```python
from build123d import *

# Parameters (mm, degrees)
BOSS_EXTRUDE1_DEPTH = 15
BOSS_EXTRUDE2_DEPTH = 7.5
SKETCH3_W           = 40
SKETCH3_H           = 75
SKETCH3_R           = 1.5
BOSS_EXTRUDE3_DEPTH = 15


with BuildPart() as part:
    # Sketch1 → Boss-Extrude1 (new body)
    with BuildSketch(Plane(origin=(0, 0, 0), x_dir=(0, 0, -1), z_dir=(1, 0, 0))):
        with BuildLine():
            Line((-37.5, 34), (-37.5, 40))
            Line((-37.5, 40), (-75, 40))
            Line((-75, 40), (-75, 0))
            Line((-75, 0), (-37.5, 0))
            Line((-37.5, 0), (-37.5, 6))
            ThreePointArc((-37.5, 6), (-51.5, 20), (-37.5, 34))
        make_face()
        with BuildLine():
            Line((0, 40), (-37.5, 40))
            Line((-37.5, 40), (-37.5, 34))
            ThreePointArc((-37.5, 34), (-27.600505063, 29.899494937), (-23.5, 20))
            ThreePointArc((-23.5, 20), (-27.600505063, 10.100505063), (-37.5, 6))
            Line((-37.5, 6), (-37.5, 0))
            Line((-37.5, 0), (0, 0))
            Line((0, 0), (0, 40))
        make_face()
    extrude(amount=BOSS_EXTRUDE1_DEPTH)

    # Sketch1_3 → Boss-Extrude2 (add)
    with BuildSketch(Plane(origin=(0, 0, 0), x_dir=(0, 0, -1), z_dir=(1, 0, 0))):
        with BuildLine():
            ThreePointArc((-23.5, 20), (-27.600505063, 29.899494937), (-37.5, 34))
            Line((-37.5, 34), (-37.5, 23))
            ThreePointArc((-37.5, 23), (-35.378679656, 22.121320344), (-34.5, 20))
            ThreePointArc((-34.5, 20), (-35.378679656, 17.878679656), (-37.5, 17))
            Line((-37.5, 17), (-37.5, 6))
            ThreePointArc((-37.5, 6), (-27.600505063, 10.100505063), (-23.5, 20))
        make_face()
        with BuildLine():
            Line((-37.5, 23), (-37.5, 34))
            ThreePointArc((-37.5, 34), (-51.5, 20), (-37.5, 6))
            Line((-37.5, 6), (-37.5, 17))
            ThreePointArc((-37.5, 17), (-40.5, 20), (-37.5, 23))
        make_face()
    extrude(amount=BOSS_EXTRUDE2_DEPTH)

    # Sketch3 → Boss-Extrude3 (add)
    with BuildSketch(Plane(origin=(0, 40, 0), x_dir=(1, 0, 0), z_dir=(0, 1, 0))):
        with Locations((20, -37.5)):
            Rectangle(SKETCH3_W, SKETCH3_H)
        with Locations(Location((8.5, -17.25, 0), (0, 0, 270))):
            Circle(SKETCH3_R, mode=Mode.SUBTRACT)
        with Locations(Location((31.5, -17.25, 0), (0, 0, 270))):
            Circle(SKETCH3_R, mode=Mode.SUBTRACT)
        with Locations(Location((31.5, -57.75, 0), (0, 0, 90))):
            Circle(SKETCH3_R, mode=Mode.SUBTRACT)
        with Locations(Location((8.5, -57.75, 0), (0, 0, 90))):
            Circle(SKETCH3_R, mode=Mode.SUBTRACT)
    extrude(amount=BOSS_EXTRUDE3_DEPTH)


solid = part.part
```
Source: CAD feature listing. Evaluate the final solid. Frame: model axes, mm. A direction names the side the tool comes from. Round coordinates to 2 decimals unless told otherwise and drop trailing zeros. Loops run counter-clockwise (first coordinate to the right, second up) from the corner with the lowest first, then second, coordinate; pieces in that order, holes last. Notation, with made-up numbers: M -25.5,-14 L -2.5,-14 A13 cw -2.5,-9 Z; hole C 2,60 d10. An arc over 180 degrees is marked long. Put each result on its own line as item: value.
(1) First-contact query: pin 1 (1 mm diameter, centred on x = 20.5, z = 61.5, fed in from -Y); pin 2 (1 mm diameter, centred on y = 20, z = 21.5, fed in from +X); pin 3 (1.5 mm diameter, centred on x = 8, z = 58, fed in from +Y). Flat tips, straight axial feed; report the tip coordinate or a pass-through.
Solutions:
pin 1: y = 40
pin 2: x = 15
pin 3: y = 40
(2) Section B-B, the plane x = 8.5. Return loops of the section in (y, z).
Solutions:
outline: M 0,0 L 55,0 L 55,15.75 L 40,15.75 L 40,18.75 L 55,18.75 L 55,56.25 L 40,56.25 L 40,59.25 L 55,59.25 L 55,75 L 0,75 Z; hole C 20,37.5 d28
(3) Section D-D, the plane z = 67. Return loops of the section in (x, y).
Solutions:
outline: M 0,0 L 15,0 L 15,40 L 40,40 L 40,55 L 0,55 Z
(4) Pull-direction query (Z, two-part tool) for faces 1 (the face through (8, 40, 17)), 2 (the face through (0, 27, 38)), 3 (the face through (11, 33, 0)), 4 (the face through (31.57, 47.4, 15.75)); classes: released by +Z, released by -Z, zero draft, split by the parting line, or undercut.
Solutions:
face 1: undercut
face 2: zero draft
face 3: released by -Z
face 4: undercut
(5) Section C-C, the plane y = 21. Return loops of the section in (x, z).
Solutions:
outline: M 0,0 L 15,0 L 15,23.54 L 7.5,23.54 L 7.5,34.67 L 0,34.67 Z; M 0,40.33 L 7.5,40.33 L 7.5,51.46 L 15,51.46 L 15,75 L 0,75 Z
(6) Access query for faces 5 (the face through (7.5, 20, 41)), 6 (the face through (15, 34, 30)), 7 (the face through (8, 40, 58)), 8 (the face through (40, 47, 38)), 9 (the face through (20, 55, 37)). Directions: +Z, -Z, +X, -X, +Y, -Y. A direction counts if a zero-diameter tool reaches every point of the face in a straight line with its end or side. Return the directions, or none.
Solutions:
face 5: +X
face 6: +Z, -Z, +X, -Y
face 7: +Y
face 8: +Z, -Z, +X, +Y, -Y
face 9: +Z, -Z, +X, -X, +Y
(7) Ray query, line 1 (X direction, y = 47.5, z = 17.25); line 2 (Z direction, x = 8, y = 48); line 3 (X direction, y = 47, z = 57). Return the intervals inside material, ascending. Write a range as [from, to].
Solutions:
line 1: [0, 7], [10, 30], [33, 40]
line 2: [0, 15.84], [18.66, 56.34], [59.16, 75]
line 3: [0, 7.2], [9.8, 30.2], [32.8, 40]
(8) Section A-A, the plane z = 57.75. Return loops of the section in (x, y), and give its area (3 significant figures).
Solutions:
outline: M 0,0 L 15,0 L 15,40 L 30,40 L 30,55 L 10,55 L 10,40 L 7,40 L 7,55 L 0,55 Z; M 33,40 L 40,40 L 40,55 L 33,55 Z
area: 1,110 mm²
